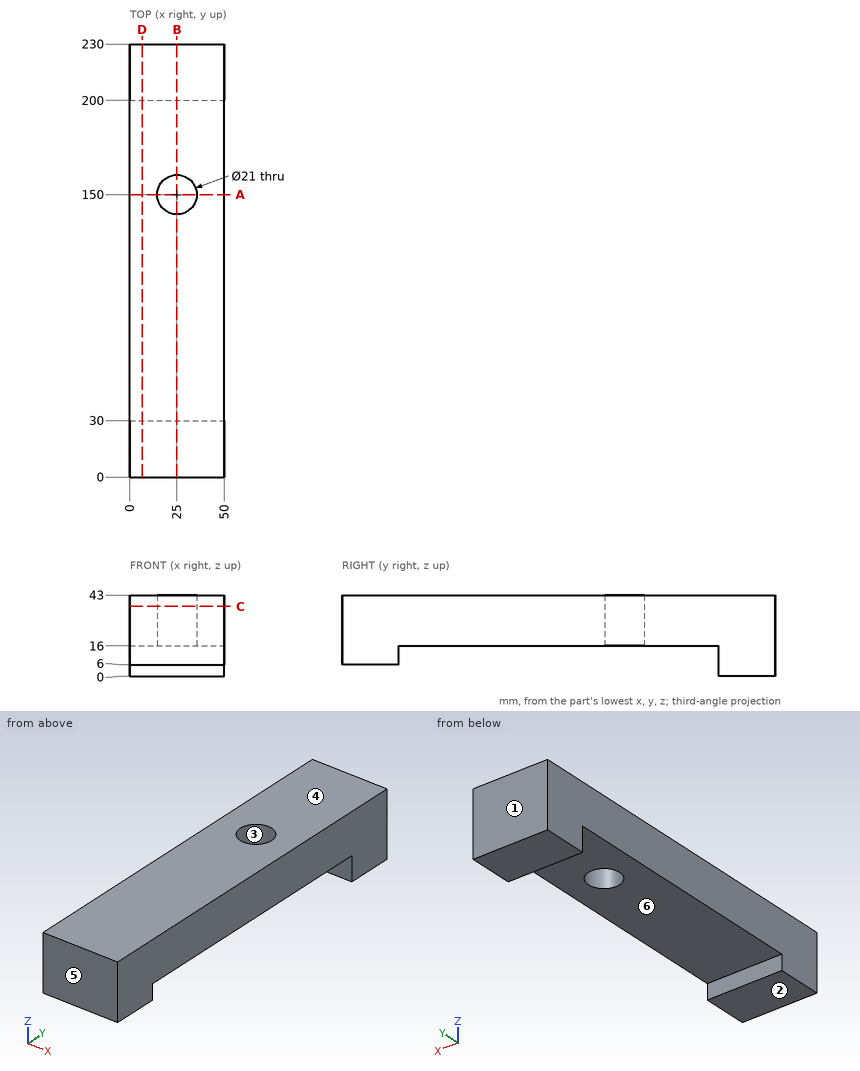
Verification items for this drawing (mm, ordinates from the low corner). A direction names the side the tool comes from. Give positions to 0.01 mm unless a question says otherwise; leave off trailing zeros. Loops run counter-clockwise (first coordinate to the right, second up) from the corner with the lowest first, then second, coordinate; pieces in that order, holes last. Notation, with made-up numbers: (59, -7.75) - (101, -7.75) arc R33 ccw to (101, 31.25) - close; hole circle Ø9 at (-25.75, 63). An arc over 180 degrees is marked (long way). Write item = value, one per line. Start each with the question number.
Q1. Tool access check on the marked faces 1 and 2. Record the directions out of +Z, -Z, +X, -X, +Y, -Y that give a thin tool (end or side, any length) a straight path to the whole face; none if there is none.
Q2. Cross-section at A-A, the plane y = 150. Enter the section's corners in (x, z), and give its area (3 significant figures).
Q3. Cross-section at B-B, the plane x = 25. Enter the section's corners in (y, z), and give its area (3 significant figures).
Q4. Thickness scan on line 1 (Y direction, x = 37, z = 10.5); line 2 (Y direction, x = 25, z = 26.5); line 3 (Z direction, x = 4, y = 154.5). Record the ranges inside material, lowest first.
Q5. Cross-section at D-D, the plane x = 6.5. Enter the section's corners in (y, z).
Q6. Cross-section at C-C, the plane z = 37. Enter the section's corners in (x, y), and give its area (3 significant figures).
Q7. Depth check by flat-ended pin: P1, Ø1.5, axis at x = 11.5, y = 182, coming from the -Z side; P2, Ø24, axis at x = 27, y = 20, coming from the -Z side. Enter the tip coordinate at first touch or a pass-through.
Q8. Mould release check, pull along Y, two halves, no side actions. Record for the marked faces 3, 4, 5 and 6: released by +Y, released by -Y, zero draft, split by the parting line, or undercut.
Answer key:
q1.face_1 = +Z, -Z, +X, -X, +Y
q1.face_2 = -Z, +X, -X, -Y
q2.outline = (0, 16) - (14.5, 16) - (14.5, 43) - (0, 43) - close; (35.5, 16) - (50, 16) - (50, 43) - (35.5, 43) - close
q2.area = 783 mm^2
q3.outline = (0, 6) - (30, 6) - (30, 16) - (139.5, 16) - (139.5, 43) - (0, 43) - close; (160.5, 16) - (200, 16) - (200, 0) - (230, 0) - (230, 43) - (160.5, 43) - close
q3.area = 6,420 mm^2
q4.line_1 = 0 to 30, 200 to 230
q4.line_2 = 0 to 139.5, 160.5 to 230
q4.line_3 = 16 to 43
q5.outline = (0, 6) - (30, 6) - (30, 16) - (200, 16) - (200, 0) - (230, 0) - (230, 43) - (0, 43) - close
q6.outline = (0, 0) - (50, 0) - (50, 230) - (0, 230) - close; hole circle Ø21 at (25, 150)
q6.area = 11,200 mm^2
q7.P1 = 16
q7.P2 = 6
q8.face_3 = undercut
q8.face_4 = zero draft
q8.face_5 = released by -Y
q8.face_6 = undercut
